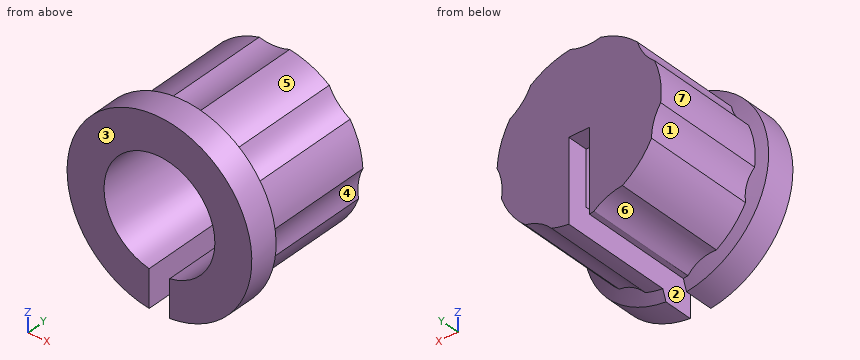
from build123d import *

# Parameters (mm, degrees)
SKETCH1_R           = 5.715
BOSS_EXTRUDE1_DEPTH = 1.778
BOSS_EXTRUDE3_DEPTH = 8.89
SKETCH6_W           = 1.27
SKETCH6_H           = 14.319161929
CUT_EXTRUDE4_DEPTH  = 13.014764004
SKETCH9_R           = 3.429
CUT_EXTRUDE6_DEPTH  = 7.62


with BuildPart() as part:
    # Sketch1 → Boss-Extrude1 (new body)
    with BuildSketch(Plane(origin=(0, 0, 0), x_dir=(1, 0, 0), z_dir=(0, 1, 0))):
        with Locations(Location((0, 0, 0), (0, 0, 270))):
            Circle(SKETCH1_R)
    extrude(amount=BOSS_EXTRUDE1_DEPTH)

    # Boss-Extrude2 cone 1 section (through the dimple's axis) → Boss-Extrude2 (revolve)
    with BuildSketch(Plane(origin=(0, 1.778, 0), x_dir=(0, 0, -1), z_dir=(1, 0, 0))):
        Polygon((0, 0), (5.715, 0), (0, 2.080089889), align=None)
    revolve(axis=Axis((0, 1.778, 0), (0, 1, 0)))

    # Sketch5 → Boss-Extrude3 (add)
    with BuildSketch(Plane.XZ):
        with BuildLine():
            ThreePointArc((3.334987409, -3.832004565), (2.446327806, -4.183135508), (1.704579152, -4.785479068))
            ThreePointArc((1.704579152, -4.785479068), (0.407862853, -5.06360029), (-0.916651171, -4.996613917))
            ThreePointArc((-0.916651171, -4.996613917), (-1.745246597, -4.520758424), (-2.678650476, -4.316391042))
            ThreePointArc((-2.678650476, -4.316391042), (-3.704583791, -3.475983161), (-4.478032723, -2.398671077))
            ThreePointArc((-4.478032723, -2.398671077), (-4.622614715, -1.45415804), (-5.044801662, -0.596972523))
            ThreePointArc((-5.044801662, -0.596972523), (-5.027403282, 0.729120186), (-4.667364299, 2.005520007))
            ThreePointArc((-4.667364299, 2.005520007), (-4.019059669, 2.707453007), (-3.612114301, 3.571978482))
            ThreePointArc((-3.612114301, 3.571978482), (-2.56448556, 4.385181161), (-1.342075361, 4.899513621))
            ThreePointArc((-1.342075361, 4.899513621), (-0.389070718, 4.830296718), (0.540568802, 5.051156835))
            ThreePointArc((0.540568802, 5.051156835), (1.829542094, 4.73911128), (2.993823697, 4.104073546))
            ThreePointArc((2.993823697, 4.104073546), (3.533896419, 3.31582848), (4.286192572, 2.726711066))
            ThreePointArc((4.286192572, 2.726711066), (4.845887235, 1.524393946), (5.075312448, 0.218182383))
            ThreePointArc((5.075312448, 0.218182383), (4.795767474, -0.695526234), (4.804225912, -1.65100375))
            ThreePointArc((4.804225912, -1.65100375), (4.213180451, -2.838223122), (3.334987409, -3.832004565))
        make_face()
    extrude(amount=-BOSS_EXTRUDE3_DEPTH)

    # Sketch6 → Cut-Extrude4 (cut, through all)
    with BuildSketch(Plane(origin=(0, 0, 0), x_dir=(-1, 0, 0), z_dir=(0, -1, 0))):
        with Locations((0, 7.159580965)):
            Rectangle(SKETCH6_W, SKETCH6_H)
    extrude(amount=-CUT_EXTRUDE4_DEPTH, mode=Mode.SUBTRACT)

    # Sketch9 → Cut-Extrude6 (cut)
    with BuildSketch(Plane.XZ):
        Circle(SKETCH9_R)
    extrude(amount=-CUT_EXTRUDE6_DEPTH, mode=Mode.SUBTRACT)


solid = part.part
Input: part model. Units: mm. Frame: model coordinates. Face numbers are marked on the shaded views. A direction names the side the tool comes from. Coordinates: 2 decimals unless noted, no trailing zeros. Loops run counter-clockwise (first coordinate to the right, second up) from the corner with the lowest first, then second, coordinate; pieces in that order, holes last.
Q1. Cut plane A-A (y = 4.25). Output: boundary loops of the cut face in (x, z) (3 decimals).
Q2. Set-up query: the marked faces 5, 6 and 7. Return all of +Z, -Z, +X, -X, +Y, -Y with unobstructed straight access to the full face (end or side cutting, diameter ignored); none if empty.
Q3. Material intervals for line 1 (Y direction, x = 1.25, z = -1.25); line 2 (X direction, y = 4, z = -1.75); line 3 (Z direction, x = 1.75, y = 6.5), sorted ascending.
Q4. Draft query along X for the marked faces 1, 2, 3 and 4. Return one class per face: +X half, -X half, draft (parallel to the pull), parting line (faces both ways), or undercut.
Q5. Contact query for flat-ended pins moving along their axis: pin 1 (3 mm diameter, centred on x = -4, y = 7.5, fed in from +Z); pin 2 (3 mm diameter, centred on y = 6, z = -0.5, fed in from +X); pin 3 (5 mm diameter, centred on y = 8, z = 2.5, fed in from -X). Output: stop coordinate, or through.
Q6. Cut plane B-B (x = 0). Output: boundary loops of the cut face in (y, z) (3 decimals).
Working result:
1. outline: (-5.045, -0.597) arc R3.137 cw to (-4.478, -2.399) arc R5.08 ccw to (-2.679, -4.316) arc R3.137 cw to (-0.917, -4.997) arc R5.08 ccw to (-0.635, -5.04) - (-0.635, -3.37) arc R3.429 cw (long way) to (0.635, -3.37) - (0.635, -5.04) arc R5.08 ccw to (1.705, -4.785) arc R3.137 cw to (3.335, -3.832) arc R5.08 ccw to (4.804, -1.651) arc R3.137 cw to (5.075, 0.218) arc R5.08 ccw to (4.286, 2.727) arc R3.137 cw to (2.994, 4.104) arc R5.08 ccw to (0.541, 5.051) arc R3.137 cw to (-1.342, 4.9) arc R5.08 ccw to (-3.612, 3.572) arc R3.137 cw to (-4.667, 2.006) arc R5.08 ccw to start
2. face 5: +Z, +X, +Y
2. face 6: -Z, -X, +Y
2. face 7: -X, +Y
3. line 1: y = 7.62 to 8.89
3. line 2: x = -4.55 to -2.95, 2.95 to 4.77
3. line 3: z = -4.74 to -2.95, 2.95 to 4.77
4. face 1: -X half
4. face 2: undercut
4. face 3: draft
4. face 4: +X half
5. pin 1: stops at z = 4.42
5. pin 2: stops at x = 5.08
5. pin 3: stops at x = -5.08
6. outline: (0, 3.429) - (7.62, 3.429) - (7.62, 0) - (8.89, 0) - (8.89, 4.886) - (2.08, 4.886) - (1.778, 5.715) - (0, 5.715) - close
